CAD build for the part. Positions are in the model's coordinates, mm. Face numbers are marked on the shaded views. A direction names the side the tool comes from. Coordinates: 2 decimals unless noted, no trailing zeros. Order: outer loops, then holes, each group sorted by start corner. A loop starts at its lowest first (then second) coordinate and runs counter-clockwise, first axis right, second up. Notation, with made-up numbers: (-18.75, 48.25) -> (-5.75, 48.25) arc R31 cw to (-5.75, 75.25) -> close; hole circle Ø8 at (30.5, 20). An arc over 180 degrees is marked (long way). Use one line per item in the form item = value. Start each with the question number.
from build123d import *

# Parameters (mm, degrees)
BOSS_EXTRUDE1_DEPTH      = 5
M3_CLEARANCE_HOLE1_D     = 3.4
M3_CLEARANCE_HOLE1_DEPTH = 5
M3_CLEARANCE_HOLE1_TIP   = 1.021463052
SKETCH4_R                = 4.725
BOSS_EXTRUDE2_DEPTH      = 33
SKETCH5_R                = 3.025
CUT_EXTRUDE1_DEPTH       = 2
FILLET1_R                = 0.5
CHAMFER1_SIZE            = 0.5
FILLET2_R                = 0.25


with BuildPart() as part:
    # Sketch1 → Boss-Extrude1 (new body)
    with BuildSketch(Plane(origin=(0, 0, 0), x_dir=(1, 0, 0), z_dir=(0, 1, 0))):
        with BuildLine():
            Line((-15, 5), (15, 5))
            ThreePointArc((15, 5), (20, 0), (15, -5))
            Line((15, -5), (-15, -5))
            ThreePointArc((-15, -5), (-20, 0), (-15, 5))
        make_face()
    extrude(amount=BOSS_EXTRUDE1_DEPTH)

    # M3 Clearance Hole1
    with Locations(Plane(origin=(0, 5, 0), x_dir=(1, 0, 0), z_dir=(0, 1, 0))):
        with Locations((-15, 0), (15, 0)):
            Hole(M3_CLEARANCE_HOLE1_D / 2, depth=M3_CLEARANCE_HOLE1_DEPTH)
            with Locations((0, 0, -(M3_CLEARANCE_HOLE1_DEPTH + M3_CLEARANCE_HOLE1_TIP / 2))):  # 118° drill point
                Cone(0, M3_CLEARANCE_HOLE1_D / 2, M3_CLEARANCE_HOLE1_TIP, mode=Mode.SUBTRACT)

    # Sketch4 → Boss-Extrude2 (add)
    with BuildSketch(Plane.XZ):
        Circle(SKETCH4_R)
    extrude(amount=BOSS_EXTRUDE2_DEPTH)

    # Sketch5 → Cut-Extrude1 (cut)
    with BuildSketch(Plane.XZ.offset(33)):
        Circle(SKETCH5_R)
    extrude(amount=-CUT_EXTRUDE1_DEPTH, mode=Mode.SUBTRACT)

    # Fillet1
    fillet1_edges = [part.edges().sort_by_distance(p)[0] for p in [
        (20, 5, 0),
        (0, 5, -5),
        (-20, 5, 0),
        (0, 0, -5),
        (20, 0, 0),
        (0, 0, 5),
        (-20, 0, 0),
        (0, 5, 5),
    ]]
    fillet(fillet1_edges, radius=FILLET1_R)

    # Chamfer1
    chamfer1_edges = [part.edges().sort_by_distance(p)[0] for p in [
        (-4.725, -33, 0),
    ]]
    chamfer(chamfer1_edges, length=CHAMFER1_SIZE)

    # Fillet2
    fillet2_edges = [part.edges().sort_by_distance(p)[0] for p in [
        (16.7, 5, 0),
        (-13.3, 5, 0),
    ]]
    fillet(fillet2_edges, radius=FILLET2_R)


solid = part.part
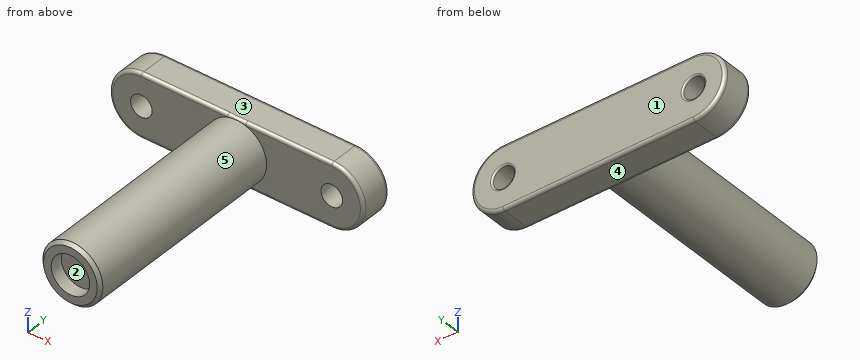
1) Two-plate mould, pull along Z, no slides. Class the marked faces 1, 2 and 3: released by +Z, released by -Z, zero draft, split by the parting line, or undercut.
2) Drop flat-ended pins along their axis: P1, Ø5, axis at x = -9, y = -21.5, coming from the +Z side; P2, Ø5, axis at y = -21, z = 1, coming from the +X side (3 decimals); P3, Ø6, axis at x = -6.5, y = -14, coming from the +Z side; P4, Ø4, axis at y = -11.5, z = 0.5, coming from the -X side (3 decimals). Give the stop position or say it passes through.
3) Cut at C-C on y = -17. Give the cut face in (x, z) (3 decimals), then the cut area to 3 significant figures.
4) Cut at A-A on z = 0. Count the separate pieces of the cut face and the enclosed holes in it, then the cut area to 3 significant figures.
5) Probe L1, parallel to X at y = 3.25, z = 0; L2, parallel to Z at x = -15, y = 3; L3, parallel to Y at x = 13.5, z = -3. List the from-to ranges inside material, lowest first.
6) 3-axis set-ups, long thin cutter, end or side, ignore diameter. For the marked faces 4 and 5: which of +Z, -Z, +X, -X, +Y, -Y reach the whole face in a straight line?
7) Cut at B-B on x = -8. Give the cut face in (y, z), then the cut area to 3 significant figures.
Values follow:
q1.face_1 = zero draft
q1.face_2 = undercut
q1.face_3 = released by +Z
q2.P1 = through
q2.P2 = 4.725
q2.P3 = 3.17
q2.P4 = -4.725
q3.outline = circle Ø9.45 at (0, 0)
q3.area = 70.1 mm^2
q4.separate_pieces = 3
q4.enclosed_holes = 0
q4.area = 465 mm^2
q5.L1 = -20 to -16.7, -13.3 to 13.3, 16.7 to 20
q5.L2 = -5 to -1.7, 1.7 to 5
q5.L3 = 0 to 5
q6.face_4 = -Z, +X, -X, +Y, -Y
q6.face_5 = -Y
q7.outline = (0, -4.5) arc R0.5 ccw to (0.5, -5) -> (4.5, -5) arc R0.5 ccw to (5, -4.5) -> (5, 4.5) arc R0.5 ccw to (4.5, 5) -> (0.5, 5) arc R0.5 ccw to (0, 4.5) -> close
q7.area = 49.8 mm^2
